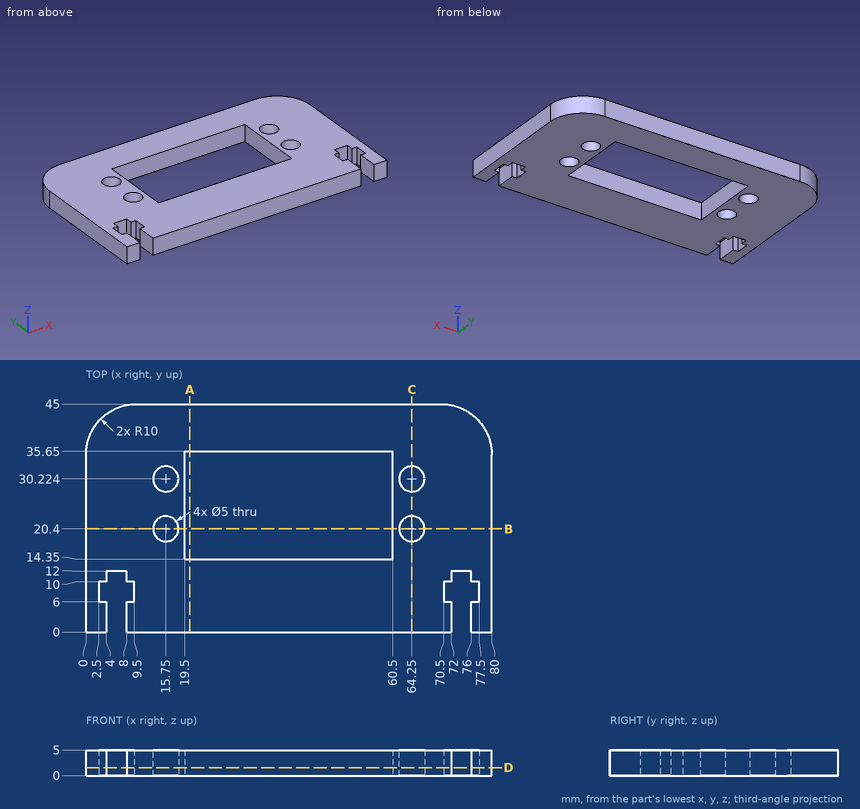
Can you work these out from the drawing? Everything is in mm from the part's minimum corner. Give positions to 0.01 mm unless a question says otherwise; leave off trailing zeros. Write each loop counter-clockwise with the first axis right and the second up, starting at its lowest first coordinate (ties: lowest second). Pieces come first, ordered by that corner, then holes. Notation, with made-up numbers: M 38.25,43.25 L 89.25,43.25 A17 cw 89.25,65.25 Z; hole C 43.5,72.25 d3. An arc over 180 degrees is marked long. Answer in a Markdown table with one row per item. Add a question column.
Item 1: Please list where these lines run through material, in increasing order: L1, parallel to Y at x = 15.75, z = 1.5; L2, parallel to X at y = 21.5, z = 0.6 (1 decimal); L3, parallel to Y at x = 36, z = 3.9.
Item 2: Imagine slicing it at C-C, the plane x = 64.25. Write out the boundary of the cut face in (y, z).
Item 3: Imagine slicing it at B-B, the plane y = 20.4. Write out the boundary of the cut face in (x, z).
Item 4: For pin 1 Ø2 at (x, z) = (73.5, 3) entering from -Y; pin 2 Ø4.5 at (x, y) = (64.25, 20.4) entering from -Z, each with a flat end and sliding along its axis, tell me the tip position at first contact or that it passes through.
Item 5: Imagine slicing it at A-A, the plane x = 20.5. Write out the boundary of the cut face in (y, z), plus the area to 4 significant figures.
Item 6: Imagine slicing it at D-D, the plane z = 1.55. State how many separate pieces and enclosed holes the cut face has.
Evaluation:
| question | item | result |
|---|---|---|
| 1 | L1 | y = 0 to 17.9, 22.9 to 27.72, 32.72 to 45 |
| 1 | L2 | x = 0 to 13.5, 18 to 19.5, 60.5 to 62, 66.5 to 80 |
| 1 | L3 | y = 0 to 14.35, 35.65 to 45 |
| 2 | outline | M 0,0 L 17.9,0 L 17.9,5 L 0,5 Z; M 22.9,0 L 27.72,0 L 27.72,5 L 22.9,5 Z; M 32.72,0 L 45,0 L 45,5 L 32.72,5 Z |
| 3 | outline | M 0,0 L 13.25,0 L 13.25,5 L 0,5 Z; M 18.25,0 L 19.5,0 L 19.5,5 L 18.25,5 Z; M 60.5,0 L 61.75,0 L 61.75,5 L 60.5,5 Z; M 66.75,0 L 80,0 L 80,5 L 66.75,5 Z |
| 4 | pin 1 | stops at y = 12 |
| 4 | pin 2 | passes through |
| 5 | outline | M 0,0 L 14.35,0 L 14.35,5 L 0,5 Z; M 35.65,0 L 45,0 L 45,5 L 35.65,5 Z |
| 5 | area | 118.5 mm² |
| 6 | separate pieces | 1 |
| 6 | enclosed holes | 5 |
